Source: CAD feature listing. Evaluate the final solid. Frame: model axes, mm. A direction names the side the tool comes from. Round coordinates to 2 decimals unless told otherwise and drop trailing zeros. Loops run counter-clockwise (first coordinate to the right, second up) from the corner with the lowest first, then second, coordinate; pieces in that order, holes last. Notation, with made-up numbers: (67, 61.25) -> (79, 61.25) arc R19 cw to (79, 95.25) -> close; hole circle Ø6 at (40.25, 54). An arc over 180 degrees is marked (long way). Return JSON: item names as keys, results as strings. Group by question number.
```python
from build123d import *

# Parameters (mm, degrees)
SKETCH2_R           = 2.15
BOSS_EXTRUDE1_DEPTH = 3


with BuildPart() as part:
    # Sketch2 → Boss-Extrude1 (new body)
    with BuildSketch(Plane.XY):
        with BuildLine():
            Line((20.505045688, 0), (5, 0))
            Line((5, 0), (5, -3.611111111))
            Line((5, -3.611111111), (2, -3.611111111))
            Line((2, -3.611111111), (2, 0))
            Line((2, 0), (0.702116043, 0))
            ThreePointArc((0.702116043, 0), (0.102828022, -0.199466511), (-0.257384219, -0.718292266))
            ThreePointArc((-0.257384219, -0.718292266), (-0.42929832, -3.650374688), (0.70215346, -6.36081352))
            ThreePointArc((0.70215346, -6.36081352), (1.058001533, -6.667450679), (1.514599965, -6.777777778))
            Line((1.514599965, -6.777777778), (22.805555556, -6.777777778))
            Line((22.805555556, -6.777777778), (24.781577826, -6.777777778))
            ThreePointArc((24.781577826, -6.777777778), (25.426089078, -6.542372603), (25.767157761, -5.94698827))
            ThreePointArc((25.767157761, -5.94698827), (24.71964165, -1.898378941), (20.993425754, 0))
            Line((20.993425754, 0), (20.505045688, 0))
        make_face()
        with Locations((22.2, -3.677777778)):
            Circle(SKETCH2_R, mode=Mode.SUBTRACT)
    extrude(amount=BOSS_EXTRUDE1_DEPTH)


solid = part.part
```
(1) Cut plane B-B (z = 1.6). Return loops of the section in (x, y).
(2) Cut plane A-A (y = -5). Return loops of the section in (x, z).
(3) Pin query (flat end, axial travel): pin 1 (3.5 mm diameter, centred on x = 22.2, y = -3.68, fed in from -Z); pin 2 (0.9 mm diameter, centred on y = -1.5, z = 1, fed in from -X); pin 3 (0.9 mm diameter, centred on y = -1, z = 1, fed in from +X). Return the tip coordinate at first contact, or that it passes through.
(4) Mould query, pull axis Y, two halves, no side actions, for faces 1 (the face through (24.25, -3.03, 1.48)), 2 (the face through (13, -6.778, 1)), 3 (the face through (-0.436, -3.609, 1.479)), 4 (the face through (1, 0, 1)). Classes: released by +Y, released by -Y, zero draft, split by the parting line, or undercut.
(5) Cut plane C-C (x = 22.2). Return loops of the section in (y, z), and give its area (3 significant figures).
(6) Ray query, line 1 (X direction, y = -3, z = 2.1); line 2 (X direction, y = -2, z = 1.5); line 3 (Y direction, x = 22.2, z = 2.2). Return the intervals inside material, ascending.
(7) Set-up query: faces 5 (the face through (5, -2, 1)), 6 (the face through (12, -3, 3)). Return all of +Z, -Z, +X, -X, +Y, -Y with unobstructed straight access to the full face (end or side cutting, diameter ignored); none if empty.
Answers follow:
{
 "1": {"outline": "(-0.26, -0.72) arc R6.53 ccw to (0.7, -6.36) arc R1 ccw to (1.51, -6.78) -> (24.78, -6.78) arc R1 ccw to (25.77, -5.95) arc R5.09 ccw to (20.99, 0) -> (5, 0) -> (5, -3.61) -> (2, -3.61) -> (2, 0) -> (0.7, 0) arc R1 ccw to start; hole circle Ø4.3 at (22.2, -3.68)"},
 "2": {"outline": "(-0.05, 0) -> (20.5, 0) -> (20.5, 3) -> (-0.05, 3) -> close; (23.9, 0) -> (25.84, 0) -> (25.84, 3) -> (23.9, 3) -> close"},
 "3": {"pin 1": "through", "pin 2": "x = -0.49", "pin 3": "x = 24.31"},
 "4": {"face 1": "undercut", "face 2": "released by -Y", "face 3": "split by the parting line", "face 4": "released by +Y"},
 "5": {"outline": "(-6.78, 0) -> (-5.83, 0) -> (-5.83, 3) -> (-6.78, 3) -> close; (-1.53, 0) -> (-0.21, 0) -> (-0.21, 3) -> (-1.53, 3) -> close", "area": "6.82 mm^2"},
 "6": {"line 1": "-0.51 to 2, 5 to 20.16, 24.24 to 25.39", "line 2": "-0.5 to 2, 5 to 20.86, 23.54 to 24.8", "line 3": "-6.78 to -5.83, -1.53 to -0.21"},
 "7": {"face 5": "+Z, -Z, +Y", "face 6": "+Z, +X, -X, +Y, -Y"}
}
